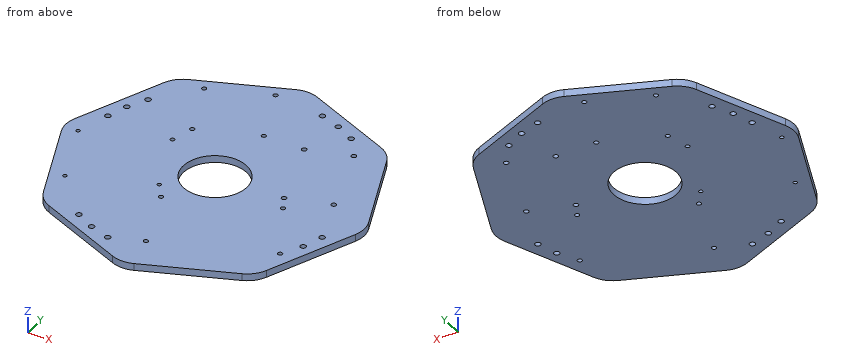
```python
from build123d import *

# Parameters (mm, degrees)
SKETCH_1_R      = 1.6
SKETCH_1_R_2    = 2
SKETCH_1_R_3    = 22.5
SKETCH_1_R_4    = 1.75
SKETCH_1_R_5    = 1.35
SKETCH_1_R_6    = 1.5
EXTRUDE_1_DEPTH = 5
FILLET_1_R      = 20


with BuildPart() as part:
    # 草图1 → 凸台-拉伸1 (new body)
    with BuildSketch(Plane.XY):
        Polygon((0, 108.239220029), (-76.536686473, 76.536686473), (-108.239220029, 0), (-76.536686473, -76.536686473), (0, -108.239220029), (76.536686473, -76.536686473), (108.239220029, 0), (76.536686473, 76.536686473), align=None)
        with Locations((0.984871452, -80.771467909)):
            Circle(SKETCH_1_R, mode=Mode.SUBTRACT)
        with Locations((77.251126861, -49.180950568)):
            Circle(SKETCH_1_R, mode=Mode.SUBTRACT)
        with Locations((-35.206875778, -84.996916991)):
            Circle(SKETCH_1_R_2, mode=Mode.SUBTRACT)
        with Locations((84.996916991, -35.206875778)):
            Circle(SKETCH_1_R_2, mode=Mode.SUBTRACT)
        with Locations((35.206875778, 84.996916991)):
            Circle(SKETCH_1_R_2, mode=Mode.SUBTRACT)
        with Locations((-84.996916991, 35.206875778)):
            Circle(SKETCH_1_R_2, mode=Mode.SUBTRACT)
        with Locations((-16.310103988, -35.699033711)):
            Circle(SKETCH_1_R, mode=Mode.SUBTRACT)
        with Locations((52.916189383, -7.024564124)):
            Circle(SKETCH_1_R, mode=Mode.SUBTRACT)
        Circle(SKETCH_1_R_3, mode=Mode.SUBTRACT)
        with Locations((-55.532225493, 76.577881479)):
            Circle(SKETCH_1_R, mode=Mode.SUBTRACT)
        with Locations((-38.694154469, 35.927182049)):
            Circle(SKETCH_1_R, mode=Mode.SUBTRACT)
        with Locations((1.956544962, 52.765253073)):
            Circle(SKETCH_1_R, mode=Mode.SUBTRACT)
        with Locations((-14.881526062, 93.415952503)):
            Circle(SKETCH_1_R, mode=Mode.SUBTRACT)
        with Locations((89.588318422, -20.926853617)):
            Circle(SKETCH_1_R_2, mode=Mode.SUBTRACT)
        with Locations((-20.926853617, -89.588318422)):
            Circle(SKETCH_1_R_2, mode=Mode.SUBTRACT)
        with Locations((-89.588318422, 20.926853617)):
            Circle(SKETCH_1_R_2, mode=Mode.SUBTRACT)
        with Locations((20.926853617, 89.588318422)):
            Circle(SKETCH_1_R_2, mode=Mode.SUBTRACT)
        with Locations((30.543151662, 53.28256885)):
            Circle(SKETCH_1_R_4, mode=Mode.SUBTRACT)
        with Locations((59.802830282, 63.216410356)):
            Circle(SKETCH_1_R_4, mode=Mode.SUBTRACT)
        with Locations((47.742521261, 2.622607486)):
            Circle(SKETCH_1_R_4, mode=Mode.SUBTRACT)
        with Locations((77.002199881, 12.556448992)):
            Circle(SKETCH_1_R_4, mode=Mode.SUBTRACT)
        with Locations((-96.543078059, -2.105725275)):
            Circle(SKETCH_1_R_5, mode=Mode.SUBTRACT)
        with Locations((-77.791589873, -47.375822368)):
            Circle(SKETCH_1_R_5, mode=Mode.SUBTRACT)
        with Locations((-42.958065173, 20.089913802)):
            Circle(SKETCH_1_R_6, mode=Mode.SUBTRACT)
        with Locations((-24.206576987, -25.180183291)):
            Circle(SKETCH_1_R_5, mode=Mode.SUBTRACT)
        with Locations((-48.55098737, -78.146027573)):
            Circle(SKETCH_1_R_2, mode=Mode.SUBTRACT)
        with Locations((-78.146027573, 48.55098737)):
            Circle(SKETCH_1_R_2, mode=Mode.SUBTRACT)
        with Locations((48.55098737, 78.146027573)):
            Circle(SKETCH_1_R_2, mode=Mode.SUBTRACT)
    extrude(amount=EXTRUDE_1_DEPTH)

    # 圆角1
    fillet_1_edges = [part.edges().sort_by_distance(p)[0] for p in [
        (76.536686473, 76.536686473, 2.5),
        (108.239220029, 0, 2.5),
        (76.536686473, -76.536686473, 2.5),
        (0, -108.239220029, 2.5),
        (-76.536686473, -76.536686473, 2.5),
        (-108.239220029, 0, 2.5),
        (-76.536686473, 76.536686473, 2.5),
        (0, 108.239220029, 2.5),
    ]]
    fillet(fillet_1_edges, radius=FILLET_1_R)


solid = part.part
```
Model file for the job. Use its own axes, mm. Round coordinates to 2 decimals unless told otherwise and drop trailing zeros. Order: outer loops, then holes, each group sorted by start corner. A loop starts at its lowest first (then second) coordinate and runs counter-clockwise, first axis right, second up. Notation, with made-up numbers: M 56,1.25 L 95,1.25 A12 ccw 95,7.25 Z; hole C 11.5,-4 d1. An arc over 180 degrees is marked long. Use CSV: the item, a comma, the result in double quotes.
Item 1: Saw through at B-B (z = 3.9). State how many separate pieces and enclosed holes the cut face has, plus the area to 3 significant figures.
Worked answers:
separate pieces,"1"
enclosed holes,"28"
area,"31,200 mm²"
Item 2: Pin check, flat tip, straight feed: pin 1 (1 mm diameter, centred on x = -56.5, z = 1, fed in from +Y). Stop position of the tip, or through.
Worked answers:
pin 1,"y = 85.04"
Item 3: Probe probe 1 along X at (y, z) = (13.5, 0.55); probe 2 along X at (y, z) = (20, 2.55); probe 3 along Y at (x, z) = (78.5, 4.3). List the from-to ranges inside material, lowest first.
Worked answers:
probe 1,"-102.65 to -18, 18 to 75.53, 78.48 to 102.65"
probe 2,"-99.95 to -91.36, -87.82 to -44.46, -41.46 to -10.31, 10.31 to 99.95"
probe 3,"-71.32 to -50.18, -48.18 to 11.65, 13.46 to 71.32"
Item 4: Saw through at A-A (y = 30). List the corners of the cut face in (x, z), plus the area to 3 significant figures.
Worked answers:
outline,"M -95.81,0 L 95.81,0 L 95.81,5 L -95.81,5 Z"
area,"958 mm²"
